Work out the finished part from the listing and answer in its coordinate system (mm). A direction names the side the tool comes from. Give positions to 0.01 mm unless a question says otherwise; leave off trailing zeros. Write each loop counter-clockwise with the first axis right and the second up, starting at its lowest first coordinate (ties: lowest second). Pieces come first, ordered by that corner, then holes. Notation, with made-up numbers: (-20.75, 5) -> (22.25, 5) arc R30 ccw to (22.25, 42) -> close; hole circle Ø5 at (85, -36.75). An arc over 180 degrees is marked (long way). Use a Markdown table: item, result. Add a question column.
Q1. Section D-D, the plane z = 27 is taken. Give the vertices of the cut face in (x, y), plus the area to 3 significant figures.
Q2. Each of these flat-tipped pins is pushed along its axis until it touches: pin 1 Ø4 at (y, z) = (18, 39.5) entering from -X; pin 2 Ø4 at (y, z) = (-23, 44.5) entering from -X; pin 3 Ø5 at (x, z) = (84, 59.5) entering from +Y. Where does it stop, or does it pass through?
Q3. Section C-C, the plane x = 32 is taken. Give the vertices of the cut face in (y, z).
Q4. For faces 4 (the face through (56, -24, 30)), 5 (the face through (78.111, 20.275, 44.65)), 6 (the face through (21, 8, 39)), determine the directions among +Z, -Z, +X, -X, +Y, -Y from which every point of the face is accessible in a straight line to the end or side of a thin tool.
Q5. Section B-B, the plane y = 0 is taken. Give the vertices of the cut face in (x, z), plus the area to 3 significant figures.
Q6. Consider line 1 (Y direction, x = -44, z = 6); line 2 (X direction, y = -0.5, z = 42); line 3 (X direction, y = 8, z = 61.5). Determine where each line is inside the solid, lowest interval first.
Q7. Section A-A, the plane z = 41 is taken. Give the vertices of the cut face in (x, y).
Q8. For a pull along Z with two mould halves and no side action, classify faces 1 (the face through (56, -24, 60)), 2 (the face through (-52.58, -42.39, 10.14)), 3 (the face through (56, 23, 60)) as pulls with the +Z half, pulls with the -Z half, needs draft (parallel to the pull), parting line crosses it, or undercut.
Autodesk Fusion 360 part; units mm, degrees
sketch "Sketch1" plane through (0, 0, 0) normal (0, 0, 1) x (1, 0, 0)
  line L0 (-56, 46) -> (56, 46)
  line L1 (56, 46) -> (56, -46)
  line L2 (56, -46) -> (-56, -46)
  line L3 (-56, -46) -> (-56, 46)
  line L4 (-56, 46) -> (56, -46) construction
  line L5 (56, 46) -> (-56, -46) construction
  dimension "d1" = 92
  dimension "d2" = 112
extrude "Extrude1" add sketch "Sketch1" along normal blind 20
sketch "Sketch2" plane through (0, 0, 0) normal (0, 0, -1) x (1, 0, 0)
  line L0 (56, 46) -> (-56, 46)
  line L1 (-56, 46) -> (-56, -46)
  line L2 (-56, -46) -> (56, -46)
  line L3 (56, -46) -> (56, 46)
  circle A0 centre (56, 0) radius 46
  dimension "d5" = 92
extrude "Extrude2" add sketch "Sketch2" against normal blind 20 contours L3 A0 picked at (67.5882, 10.0412)
sketch "Sketch3" plane through (0, 0, 20) normal (0, 0, 1) x (-1, 0, 0)
  line L0 (56, 46) -> (-56, 46)
  arc A0 (-56, 46) -> (-56, -46) centre (-56, 0) ccw
  line L1 (-56, -46) -> (56, -46)
  line L2 (56, -46) -> (56, 46)
  circle A1 centre (-56, 0) radius 30
  dimension "d8" = 60
extrude "Extrude3" add sketch "Sketch3" along normal blind 50 contours A1
ref_plane "WorkPlane1" through (56, -30, 48.1933) normal (0, -1, 0) x (-1, 0, 0)
sketch "Sketch4" plane through (56, -30, 48.1933) normal (0, -1, 0) x (1, 0, 0)
  line L0 (30, 21.8067) -> (-30, 21.8067)
  line L1 (0, -48.1933) -> (46, -48.1933)
  line L2 (46, -28.1933) -> (30, -28.1933)
  line L3 (-112, -48.1933) -> (-112, -28.1933)
  line L4 (-112, -48.1933) -> (0, -48.1933)
  line L5 (-30, -28.1933) -> (-112, -28.1933)
  line L6 (30, -28.1933) -> (30, 21.8067)
  line L7 (-30, -28.1933) -> (-30, 21.8067)
  line L8 (46, -48.1933) -> (46, -28.1933)
  line L9 (0, 21.8067) -> (0, 11.8067) construction
  line L10 (0, 11.8067) -> (0, -3.1933) construction
  line L11 (15, 11.8067) -> (-15, 11.8067)
  line L12 (-15, 11.8067) -> (-15, -18.1933)
  line L13 (-15, -18.1933) -> (15, -18.1933)
  line L14 (15, -18.1933) -> (15, 11.8067)
  line L15 (15, 11.8067) -> (-15, -18.1933) construction
  line L16 (-15, 11.8067) -> (15, -18.1933) construction
  point P0 (0, -3.1933)
  dimension "d12" = 10
  dimension "d13" = 15
  dimension "d14" = 30
  dimension "d15" = 30
extrude "Extrude4" cut sketch "Sketch4" against normal blind 100 contours L11 L12 L13 L14
sketch "Sketch5" plane through (0, 0, 70) normal (0, 0, 1) x (-1, 0, 0)
  circle A0 centre (-56, 0) radius 30
  circle A1 centre (-56, 0) radius 20
  dimension "d18" = 40
extrude "Extrude5" cut sketch "Sketch5" against normal blind 120 contours A1
sketch "Sketch6" plane through (0, 0, 20) normal (0, 0, 1) x (-1, 0, 0)
  circle A0 centre (-56, 0) radius 30
  line L0 (56, 46) -> (-56, 46)
  arc A1 (-56, 46) -> (-56, -46) centre (-56, 0) ccw
  line L1 (-56, -46) -> (56, -46)
  line L2 (56, -46) -> (56, 46)
  line L3 (56, -46) -> (56, -34) construction
  line L4 (56, -34) -> (44, -34) construction
  circle A2 centre (44, -34) radius 12
  line L5 (56, 46) -> (56, 34) construction
  line L6 (56, 34) -> (44, 34) construction
  circle A3 centre (44, 34) radius 12
  circle A4 centre (44, 34) radius 6
  circle A5 centre (44, -34) radius 6
  dimension "d21" = 12
  dimension "d22" = 12
  dimension "d23" = 24
  dimension "d24" = 12
  dimension "d25" = 12
  dimension "d26" = 24
  dimension "d27" = 12
  dimension "d28" = 12
extrude "Extrude6" cut sketch "Sketch6" against normal blind 30 contours A4 | A5
sketch "Sketch7" plane through (0, 0, 20) normal (0, 0, 1) x (-1, 0, 0)
  circle A0 centre (44, -34) radius 6
  circle A1 centre (44, 34) radius 6
  circle A2 centre (-56, 0) radius 30
  line L0 (56, 46) -> (-56, 46)
  arc A3 (-56, 46) -> (-56, -46) centre (-56, 0) ccw
  line L1 (-56, -46) -> (56, -46)
  line L2 (56, -46) -> (56, 46)
  circle A4 centre (44, -34) radius 12
  circle A5 centre (44, 34) radius 12
  dimension "d31" = 24
  dimension "d32" = 24
extrude "Extrude7" cut sketch "Sketch7" against normal blind 40 contours L0 L2 A5 | L1 L2 A4
sketch "Sketch8" plane through (0, 0, 20) normal (0, 0, 1) x (-1, 0, 0)
  arc A0 (56, 34) -> (44, 46) centre (44, 34) ccw
  line L0 (44, 46) -> (-56, 46)
  arc A1 (-56, 46) -> (-56, -46) centre (-56, 0) ccw
  line L1 (-56, -46) -> (44, -46)
  arc A2 (44, -46) -> (56, -34) centre (44, -34) ccw
  line L2 (56, -34) -> (56, 34)
  circle A3 centre (44, -34) radius 6
  circle A4 centre (44, 34) radius 6
  circle A5 centre (-56, 0) radius 30
  line L3 (44, -34) -> (9, -34) construction
  line L4 (9, 34) -> (9, 0) construction
  line L5 (9, -27) -> (32.3827, -13.5)
  line L6 (32.3827, -13.5) -> (32.3827, 13.5)
  line L7 (32.3827, 13.5) -> (9, 27)
  line L8 (9, 27) -> (-14.3827, 13.5)
  line L9 (-14.3827, 13.5) -> (-14.3827, -13.5)
  line L10 (-14.3827, -13.5) -> (9, -27)
  line L11 (9, -34) -> (9, -27)
  arc A6 (-14.3827, -11.3688) -> (-12.537, -14.5656) centre (9, 0) ccw construction
  arc A7 (-12.537, 14.5656) -> (-14.3827, 11.3688) centre (9, 0) ccw construction
  arc A8 (10.8457, 25.9344) -> (7.1543, 25.9344) centre (9, 0) ccw construction
  arc A9 (10.8457, -25.9344) -> (32.3827, -11.3688) centre (9, 0) ccw construction
  arc A10 (32.3827, 11.3688) -> (30.537, 14.5656) centre (9, 0) ccw construction
  point P0 (9, 0)
  dimension "d35" = 35
  dimension "d36" = 52
extrude "Extrude8" add sketch "Sketch8" along normal blind 50 contours L5 L6 L7 L8 L9 L10
sketch "Sketch9" plane through (0, 0, 20) normal (0, 0, 1) x (-1, 0, 0)
  line L0 (-14.3827, -13.5) -> (-14.3827, 13.5)
  line L1 (-14.3827, 13.5) -> (9, 27)
  line L2 (9, 27) -> (32.3827, 13.5)
  line L3 (32.3827, 13.5) -> (32.3827, -13.5)
  line L4 (32.3827, -13.5) -> (9, -27)
  line L5 (9, -27) -> (-14.3827, -13.5)
  arc A0 (56, 34) -> (44, 46) centre (44, 34) ccw
  line L6 (44, 46) -> (-56, 46)
  arc A1 (-56, 46) -> (-56, -46) centre (-56, 0) ccw
  line L7 (-56, -46) -> (44, -46)
  arc A2 (44, -46) -> (56, -34) centre (44, -34) ccw
  line L8 (56, -34) -> (56, 34)
  circle A3 centre (44, -34) radius 6
  circle A4 centre (44, 34) radius 6
  circle A5 centre (-56, 0) radius 30
  line L9 (-14.3827, -13.5) -> (9, -27)
  line L10 (9, -27) -> (32.3827, -13.5)
  line L11 (32.3827, -13.5) -> (32.3827, 13.5)
  line L12 (32.3827, 13.5) -> (9, 27)
  line L13 (9, 27) -> (-14.3827, 13.5)
  line L14 (-14.3827, 13.5) -> (-14.3827, -13.5)
  circle A6 centre (-56, 0) radius 20
  circle A7 centre (-56, 0) radius 30
  line L15 (-10, 0) -> (-29.7237, 0) construction
  line L16 (-10, 0) -> (-10, -8) construction
  line L17 (-10, -8) -> (-32.4254, -8)
  line L18 (-32.4254, -8) -> (-32.4254, 8)
  line L19 (-32.4254, 8) -> (-10, 8)
  line L20 (-10, 8) -> (-10, -8)
  dimension "d39" = 8
  dimension "d40" = 16
extrude "Extrude9" add sketch "Sketch9" along normal blind 38 contours L0 A5 L14 A7 L17 L19 | L0 L14 L17 L19 L20 | A5 A7 L17 L18 L19 picked at (-30.2836, 0)
equation "d1 = 68 mm + 12 mm + 12 mm"
equation "d5 = 46 mm + 46 mm"
equation "d41 = 50 mm - 12 mm"
Result set:
| question | item | result |
|---|---|---|
| 1 | outline | (-32.38, -13.5) -> (-9, -27) -> (14.38, -13.5) -> (14.38, -8) -> (27.09, -8) arc R30 ccw (long way) to (27.09, 8) -> (14.38, 8) -> (14.38, 13.5) -> (-9, 27) -> (-32.38, 13.5) -> close; hole circle Ø40 at (56, 0) |
| 1 | area | 3,660 mm2 |
| 2 | pin 1 | stops at x = -28.05 |
| 2 | pin 2 | stops at x = -19.39 |
| 2 | pin 3 | stops at y = 15.8 |
| 3 | outline | (-46, 0) -> (46, 0) -> (46, 20) -> (18, 20) -> (18, 70) -> (-18, 70) -> (-18, 20) -> (-46, 20) -> close |
| 4 | face 4 | +Y, -Y |
| 4 | face 5 | +Z |
| 4 | face 6 | +Z, +Y |
| 5 | outline | (-56, 0) -> (36, 0) -> (36, 70) -> (26, 70) -> (26, 58) -> (14.38, 58) -> (14.38, 70) -> (-32.38, 70) -> (-32.38, 20) -> (-56, 20) -> close; (76, 0) -> (102, 0) -> (102, 20) -> (86, 20) -> (86, 70) -> (76, 70) -> close |
| 5 | area | 6,140 mm2 |
| 6 | line 1 | y = -46 to -40, -28 to 28, 40 to 46 |
| 6 | line 2 | x = -32.38 to 36.01, 75.99 to 86 |
| 6 | line 3 | x = -32.38 to 14.38, 27.09 to 37.67, 74.33 to 84.91 |
| 7 | outline | (-32.38, -13.5) -> (-9, -27) -> (14.38, -13.5) -> (14.38, -8) -> (27.09, -8) arc R30 ccw to (41, -25.98) -> (41, -13.23) arc R20 cw to (41, 13.23) -> (41, 25.98) arc R30 ccw to (27.09, 8) -> (14.38, 8) -> (14.38, 13.5) -> (-9, 27) -> (-32.38, 13.5) -> close; (71, -25.98) arc R30 ccw to (71, 25.98) -> (71, 13.23) arc R20 cw to (71, -13.23) -> close |
| 8 | face 1 | undercut |
| 8 | face 2 | needs draft |
| 8 | face 3 | undercut |
